```python
from build123d import *

# Parameters (mm, degrees)
BOSS_EXTRUDE1_DEPTH = 36
SKETCH2_R           = 1.25
CUT_EXTRUDE1_DEPTH  = 55.829280499
CHAMFER1_SIZE       = 3
SKETCH4_R           = 8
BOSS_EXTRUDE2_DEPTH = 40
FILLET1_R           = 10
SKETCH5_W           = 25
SKETCH5_H           = 10
CUT_EXTRUDE3_DEPTH  = 49.176757882
CHAMFER2_SIZE       = 2


with BuildPart() as part:
    # Sketch1 → Boss-Extrude1 (new body)
    with BuildSketch(Plane.XY):
        Polygon((-10.5, 17), (-3, 17), (-3, -17), (-10.5, -17), (-10.5, -20), (0, -20), (0, 20), (-10.5, 20), align=None)
    extrude(amount=BOSS_EXTRUDE1_DEPTH)

    # Sketch2 → Cut-Extrude1 (cut, through all)
    with BuildSketch(Plane(origin=(0, 20, 0), x_dir=(1, 0, 0), z_dir=(0, 1, 0))):
        with Locations(Location((-7.7, -3.5, 0), (0, 0, 270))):
            Circle(SKETCH2_R)
        with Locations(Location((-7.7, -25.5, 0), (0, 0, 270))):
            Circle(SKETCH2_R)
    extrude(amount=-CUT_EXTRUDE1_DEPTH, mode=Mode.SUBTRACT)

    # Chamfer1
    chamfer1_edges = [part.edges().sort_by_distance(p)[0] for p in [
        (-10.5, 18.5, 0),
        (-10.5, -18.5, 36),
        (-10.5, 18.5, 36),
        (-10.5, -18.5, 0),
    ]]
    chamfer(chamfer1_edges, length=CHAMFER1_SIZE)

    # Sketch4 → Boss-Extrude2 (add, through all)
    with BuildSketch(Plane(origin=(0, 20, 0), x_dir=(1, 0, 0), z_dir=(0, 1, 0))):
        with BuildLine():
            Line((13, -7.5), (0, -7.5))
            Line((0, -7.5), (0, -31.5))
            Line((0, -31.5), (13, -31.5))
            ThreePointArc((13, -31.5), (25, -19.5), (13, -7.5))
        make_face()
        with Locations(Location((13, -19.5, 0), (0, 0, 270))):
            Circle(SKETCH4_R, mode=Mode.SUBTRACT)
    extrude(amount=-BOSS_EXTRUDE2_DEPTH)

    # Fillet1
    # the kernel refuses this fillet: 10 mm, written as the material it adds along each edge
    with BuildSketch(Plane(origin=(0, 20, 7.5), x_dir=(0, 0, -1), z_dir=(0, -1, 0))) as fillet1_piece_1:
        with BuildLine():
            CenterArc((10, 9.682458366), FILLET1_R, 180, 75.522487814)
            Line((0, 9.682458366), (-0.2, 9.682458366))
            Line((-0.2, 9.682458366), (-0.2, 0))
            Line((-0.2, 0), (0, -0.2))
            ThreePointArc((0, -0.2), (3.75, -0.2), (7.45, -0.193649167))
            Line((7.45, -0.193649167), (7.5, 0))
        make_face()
    extrude(amount=40)
    with BuildSketch(Plane(origin=(0, 20, 31.5), x_dir=(1.5375725384245926e-12, 0, 1.0), z_dir=(0, -1, 0))) as fillet1_piece_2:
        with BuildLine():
            CenterArc((10, -8.351646544), FILLET1_R, 123.367012969, 56.632987031)
            Line((0, -8.351646544), (-0.2, -8.351646544))
            Line((-0.2, -8.351646544), (-0.2, 0))
            Line((-0.2, 0), (0, 0.2))
            ThreePointArc((0, 0.2), (2.25, 0.2), (4.39, 0.167032931))
            Line((4.39, 0.167032931), (4.5, 0))
        make_face()
    extrude(amount=40)

    # Sketch5 → Cut-Extrude3 (cut, through all)
    with BuildSketch(Plane.XY.offset(36)):
        with Locations((12.5, 15)):
            Rectangle(SKETCH5_W, SKETCH5_H)
        with Locations((12.5, -15)):
            Rectangle(SKETCH5_W, SKETCH5_H)
    extrude(amount=-CUT_EXTRUDE3_DEPTH, mode=Mode.SUBTRACT)

    # Chamfer2
    chamfer2_edges = [part.edges().sort_by_distance(p)[0] for p in [
        (0, 20, 18),
        (0, -20, 18),
    ]]
    chamfer(chamfer2_edges, length=CHAMFER2_SIZE)


solid = part.part
```
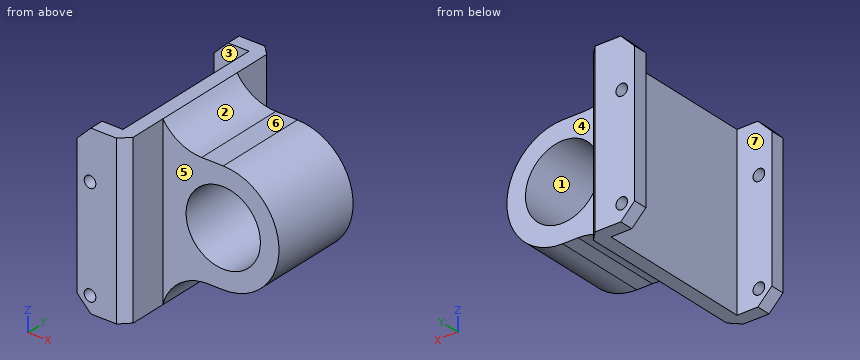
Input: part model. Units: mm. Frame: model coordinates. Face numbers are marked on the shaded views. A direction names the side the tool comes from. Round coordinates to 2 decimals unless told otherwise and drop trailing zeros. Order: outer loops, then holes, each group sorted by start corner. A loop starts at its lowest first (then second) coordinate and runs counter-clockwise, first axis right, second up. Notation, with made-up numbers: (30, -37.75) - (40, -37.75) arc R9 ccw to (40, -33.75) - close; hole circle Ø9 at (-17, 15). An arc over 180 degrees is marked (long way). Answer in a Markdown table with one row per item.
Item 1: Section query A-A (z = 19.5). Return the cut outline in (x, y).
Model answer:
| item | result |
|---|---|
| outline | (-10.5, -20) - (-2, -20) - (0, -18) - (0, -10) - (5, -10) - (5, 10) - (0, 10) - (0, 18) - (-2, 20) - (-10.5, 20) - (-10.5, 17) - (-3, 17) - (-3, -17) - (-10.5, -17) - close; (21, -10) - (25, -10) - (25, 10) - (21, 10) - close |
Item 2: Line query: line 1 (X direction, y = 1, z = 19.5); line 2 (Z direction, x = -7, y = -18); line 3 (Y direction, x = -8, z = 19). Output: solid intervals per line, ascending.
Model answer:
| item | result |
|---|---|
| line 1 | x = -3 to 5, 21 to 25 |
| line 2 | z = 0 to 2.46, 4.54 to 24.46, 26.54 to 36 |
| line 3 | y = -20 to -17, 17 to 20 |
Item 3: Section query B-B (y = 3). Return the cut outline in (x, z), then the cut area to 3 significant figures.
Model answer:
| item | result |
|---|---|
| outline | (-3, 0) - (0, 0) arc R10 cw to (9.68, 7.5) - (13, 7.5) arc R12 ccw to (13, 31.5) - (8.35, 31.5) arc R10 cw to (0, 36) - (-3, 36) - close; hole circle Ø16 at (13, 19.5) |
| area | 475 mm² |
Item 4: Pin query (flat end, axial travel): pin 1 (1.5 mm diameter, centred on y = 9, z = 8, fed in from +X); pin 2 (1.5 mm diameter, centred on x = -7.7, z = 25.5, fed in from +Y); pin 3 (4 mm diameter, centred on y = 14.5, z = 16, fed in from +X); pin 4 (1 mm diameter, centred on x = 5.5, z = 27, fed in from -Y). Return the tip coordinate at first contact, or that it passes through.
Model answer:
| item | result |
|---|---|
| pin 1 | stops at x = 18.33 |
| pin 2 | passes through |
| pin 3 | stops at x = 0 |
| pin 4 | stops at y = -10 |
Item 5: Mould query, pull axis X, two halves, no side actions, for the marked faces 1, 2 and 3. Classes: released by +X, released by -X, zero draft, split by the parting line, or undercut.
Model answer:
| item | result |
|---|---|
| face 1 | undercut |
| face 2 | released by +X |
| face 3 | zero draft |
Item 6: Section query D-D (z = 23.5). Return the cut outline in (x, y), then the cut area to 3 significant figures.
Model answer:
| item | result |
|---|---|
| outline | (-10.5, -20) - (-2, -20) - (0, -18) - (0, -10) - (6.07, -10) - (6.07, 10) - (0, 10) - (0, 18) - (-2, 20) - (-10.5, 20) - (-10.5, 17) - (-3, 17) - (-3, -17) - (-10.5, -17) - close; (19.93, -10) - (24.31, -10) - (24.31, 10) - (19.93, 10) - close |
| area | 370 mm² |
Item 7: Reachability of the marked faces 4, 5, 6 and 7 from +Z, -Z, +X, -X, +Y, -Y: full face, straight path, thin tool, end or side. Return the list, or none.
Model answer:
| item | result |
|---|---|
| face 4 | +Z, -Z, +X, +Y |
| face 5 | +Z, -Z, +X, -Y |
| face 6 | +Z, +X, +Y, -Y |
| face 7 | +Z, -Z, -X |
Item 8: Section query C-C (x = 16). Return the cut outline in (y, z), then the cut area to 3 significant figures.
Model answer:
| item | result |
|---|---|
| outline | (-10, 7.88) - (10, 7.88) - (10, 12.08) - (-10, 12.08) - close; (-10, 26.92) - (10, 26.92) - (10, 31.12) - (-10, 31.12) - close |
| area | 168 mm² |
